Can you work these out from the model? Positions are in its coordinate system, mm. A direction names the side the tool comes from. Give positions to 0.01 mm unless a question says otherwise; leave off trailing zeros. Write each loop counter-clockwise with the first axis right and the second up, starting at its lowest first coordinate (ties: lowest second). Pieces come first, ordered by that corner, then holes.
from build123d import *

# Parameters (mm, degrees)
F0_R     = 45.212
F0_R_2   = 2.032
F1_DEPTH = 6.35
F2_DEPTH = 10.16


with BuildPart() as f1:
    # F0 (on Front) → F1 (new body)
    with BuildSketch(Plane.XZ):
        Circle(F0_R)
        with BuildLine():
            ThreePointArc((37.1053751064, 15.2894918888), (39.3680729638, 7.7930902161), (40.132, 0))
            ThreePointArc((40.132, 0), (39.3680729638, -7.7930902161), (37.1053751064, -15.2894918888))
            ThreePointArc((37.1053751064, -15.2894918888), (34.7553315047, -20.066), (31.7937759398, -24.4894515147))
            ThreePointArc((31.7937759398, -24.4894515147), (20.066, -34.7553315047), (5.3115991666, -39.7789434034))
            ThreePointArc((5.3115991666, -39.7789434034), (0, -40.132), (-5.3115991666, -39.7789434034))
            ThreePointArc((-5.3115991666, -39.7789434034), (-20.066, -34.7553315047), (-31.7937759398, -24.4894515147))
            ThreePointArc((-31.7937759398, -24.4894515147), (-34.7553315047, -20.066), (-37.1053751064, -15.2894918888))
            ThreePointArc((-37.1053751064, -15.2894918888), (-40.132, 0), (-37.1053751064, 15.2894918888))
            ThreePointArc((-37.1053751064, 15.2894918888), (-34.7553315047, 20.066), (-31.7937759398, 24.4894515147))
            ThreePointArc((-31.7937759398, 24.4894515147), (-20.066, 34.7553315047), (-5.3115991666, 39.7789434034))
            ThreePointArc((-5.3115991666, 39.7789434034), (0, 40.132), (5.3115991666, 39.7789434034))
            ThreePointArc((5.3115991666, 39.7789434034), (20.066, 34.7553315047), (31.7937759398, 24.4894515147))
            ThreePointArc((31.7937759398, 24.4894515147), (34.7553315047, 20.066), (37.1053751064, 15.2894918888))
        make_face(mode=Mode.SUBTRACT)
        Polygon((4.2527620829, -7.366), (8.5055241657, 0), (4.2527620829, 7.366), (-4.2527620829, 7.366), (-8.5055241657, 0), (-4.2527620829, -7.366), align=None)
        Circle(F0_R_2, mode=Mode.SUBTRACT)
        with BuildLine():
            Line((1.5875, 35.4173183441), (5.3115991666, 39.7789434034))
            ThreePointArc((5.3115991666, 39.7789434034), (0, 40.132), (-5.3115991666, 39.7789434034))
            Line((-5.3115991666, 39.7789434034), (-1.5875, 35.4173183441))
            Line((-1.5875, 35.4173183441), (-1.5875, 12.7893453464))
            Line((-1.5875, 12.7893453464), (-5.4585231293, 9.4544393942))
            Line((-5.4585231293, 9.4544393942), (5.4585231293, 9.4544393942))
            Line((5.4585231293, 9.4544393942), (1.5875, 12.7893453464))
            Line((1.5875, 12.7893453464), (1.5875, 35.4173183441))
        make_face()
        with BuildLine():
            Line((-29.8785474199, 19.0834745006), (-31.7937759398, 24.4894515147))
            ThreePointArc((-31.7937759398, 24.4894515147), (-34.7553315047, 20.066), (-37.1053751064, 15.2894918888))
            Line((-37.1053751064, 15.2894918888), (-31.4660474199, 16.3338438436))
            Line((-31.4660474199, 16.3338438436), (-11.8696479677, 5.0198573447))
            Line((-11.8696479677, 5.0198573447), (-10.9170462585, 0))
            Line((-10.9170462585, 0), (-5.4585231293, 9.4544393942))
            Line((-5.4585231293, 9.4544393942), (-10.2821479677, 7.7694880017))
            Line((-10.2821479677, 7.7694880017), (-29.8785474199, 19.0834745006))
        make_face()
        with BuildLine():
            ThreePointArc((-37.1053751064, -15.2894918888), (-34.7553315047, -20.066), (-31.7937759398, -24.4894515147))
            Line((-31.7937759398, -24.4894515147), (-29.8785474199, -19.0834745006))
            Line((-29.8785474199, -19.0834745006), (-10.2821479677, -7.7694880017))
            Line((-10.2821479677, -7.7694880017), (-5.4585231293, -9.4544393942))
            Line((-5.4585231293, -9.4544393942), (-10.9170462585, 0))
            Line((-10.9170462585, 0), (-11.8696479677, -5.0198573447))
            Line((-11.8696479677, -5.0198573447), (-31.4660474199, -16.3338438436))
            Line((-31.4660474199, -16.3338438436), (-37.1053751064, -15.2894918888))
        make_face()
        with BuildLine():
            ThreePointArc((-5.3115991666, -39.7789434034), (0, -40.132), (5.3115991666, -39.7789434034))
            Line((5.3115991666, -39.7789434034), (1.5875, -35.4173183441))
            Line((1.5875, -35.4173183441), (1.5875, -12.7893453464))
            Line((1.5875, -12.7893453464), (5.4585231293, -9.4544393942))
            Line((5.4585231293, -9.4544393942), (-5.4585231293, -9.4544393942))
            Line((-5.4585231293, -9.4544393942), (-1.5875, -12.7893453464))
            Line((-1.5875, -12.7893453464), (-1.5875, -35.4173183441))
            Line((-1.5875, -35.4173183441), (-5.3115991666, -39.7789434034))
        make_face()
        with BuildLine():
            ThreePointArc((31.7937759398, -24.4894515147), (34.7553315047, -20.066), (37.1053751064, -15.2894918888))
            Line((37.1053751064, -15.2894918888), (31.4660474199, -16.3338438436))
            Line((31.4660474199, -16.3338438436), (11.8696479677, -5.0198573447))
            Line((11.8696479677, -5.0198573447), (10.9170462585, 0))
            Line((10.9170462585, 0), (5.4585231293, -9.4544393942))
            Line((5.4585231293, -9.4544393942), (10.2821479677, -7.7694880017))
            Line((10.2821479677, -7.7694880017), (29.8785474199, -19.0834745006))
            Line((29.8785474199, -19.0834745006), (31.7937759398, -24.4894515147))
        make_face()
        with BuildLine():
            Line((31.4660474199, 16.3338438436), (37.1053751064, 15.2894918888))
            ThreePointArc((37.1053751064, 15.2894918888), (34.7553315047, 20.066), (31.7937759398, 24.4894515147))
            Line((31.7937759398, 24.4894515147), (29.8785474199, 19.0834745006))
            Line((29.8785474199, 19.0834745006), (10.2821479677, 7.7694880017))
            Line((10.2821479677, 7.7694880017), (5.4585231293, 9.4544393942))
            Line((5.4585231293, 9.4544393942), (10.9170462585, 0))
            Line((10.9170462585, 0), (11.8696479677, 5.0198573447))
            Line((11.8696479677, 5.0198573447), (31.4660474199, 16.3338438436))
        make_face()
        Polygon((-4.2527620829, 7.366), (-5.4585231293, 9.4544393942), (-10.9170462585, 0), (-8.5055241657, 0), align=None)
        Polygon((-10.9170462585, 0), (-5.4585231293, -9.4544393942), (-4.2527620829, -7.366), (-8.5055241657, 0), align=None)
        Polygon((-5.4585231293, -9.4544393942), (5.4585231293, -9.4544393942), (4.2527620829, -7.366), (-4.2527620829, -7.366), align=None)
        Polygon((5.4585231293, -9.4544393942), (10.9170462585, 0), (8.5055241657, 0), (4.2527620829, -7.366), align=None)
        Polygon((8.5055241657, 0), (10.9170462585, 0), (5.4585231293, 9.4544393942), (4.2527620829, 7.366), align=None)
        Polygon((4.2527620829, 7.366), (5.4585231293, 9.4544393942), (-5.4585231293, 9.4544393942), (-4.2527620829, 7.366), align=None)
    extrude(amount=F1_DEPTH)

    # F0 (on Front) → F2 (join)
    with BuildSketch(Plane.XZ):
        Polygon((-10.9170462585, 0), (-5.4585231293, -9.4544393942), (-4.2527620829, -7.366), (-8.5055241657, 0), align=None)
        Polygon((-5.4585231293, -9.4544393942), (5.4585231293, -9.4544393942), (4.2527620829, -7.366), (-4.2527620829, -7.366), align=None)
        Polygon((5.4585231293, -9.4544393942), (10.9170462585, 0), (8.5055241657, 0), (4.2527620829, -7.366), align=None)
        Polygon((8.5055241657, 0), (10.9170462585, 0), (5.4585231293, 9.4544393942), (4.2527620829, 7.366), align=None)
        Polygon((4.2527620829, 7.366), (5.4585231293, 9.4544393942), (-5.4585231293, 9.4544393942), (-4.2527620829, 7.366), align=None)
        Polygon((-4.2527620829, 7.366), (-5.4585231293, 9.4544393942), (-10.9170462585, 0), (-8.5055241657, 0), align=None)
    extrude(amount=F2_DEPTH)


solid = f1.part
(1) Imagine slicing it at B-B, the plane x = 22. Write out the boundary of the cut face in (y, z), plus the area to 3 significant figures.
Returned:
outline: (-6.35, -39.5) - (0, -39.5) - (0, -33.56) - (-6.35, -33.56) - close; (-6.35, -14.53) - (0, -14.53) - (0, -10.87) - (-6.35, -10.87) - close; (-6.35, 10.87) - (0, 10.87) - (0, 14.53) - (-6.35, 14.53) - close; (-6.35, 33.56) - (0, 33.56) - (0, 39.5) - (-6.35, 39.5) - close
area: 122 mm2
(2) If I drill on L1, parallel to Z at x = 0, y = -3; L2, parallel to Z at x = 3, y = -0.25; L3, parallel to Z at x = 23, y = -6.25, over which ranges is the centre line in solid material (lowest first)?
Returned:
L1: z = -45.21 to -2.03, 2.03 to 45.21
L2: z = -45.11 to -37.07, -11.57 to 11.57, 37.07 to 45.11
L3: z = -38.92 to -32.89, -15.11 to -11.45, 11.45 to 15.11, 32.89 to 38.92
(3) Imagine slicing it at A-A, the plane x = 0. Write out the boundary of the cut face in (y, z).
Returned:
outline: (-10.16, -9.45) - (-6.35, -9.45) - (-6.35, -45.21) - (0, -45.21) - (0, -2.03) - (-6.35, -2.03) - (-6.35, -7.37) - (-10.16, -7.37) - close; (-10.16, 7.37) - (-6.35, 7.37) - (-6.35, 2.03) - (0, 2.03) - (0, 45.21) - (-6.35, 45.21) - (-6.35, 9.45) - (-10.16, 9.45) - close
(4) Will these pins go through, and if not, where does the flat tip stop? P1, Ø2, axis at x = 20.5, y = -6.5, coming from the -Z side; P2, Ø3, axis at y = -4, z = -29, coming from the -X side; P3, Ø1.9, axis at y = -4, z = 20.5, coming from the -X side.
Returned:
P1: stops at z = -40.79
P2: stops at x = -35.89
P3: stops at x = -40.77
(5) Imagine slicing it at C-C, the plane z = -38. Write out the boundary of the cut face in (x, y), plus the area to 3 significant figures.
Returned:
outline: (-24.5, -6.35) - (-12.91, -6.35) - (-12.91, 0) - (-24.5, 0) - close; (-3.79, -6.35) - (3.79, -6.35) - (3.79, 0) - (-3.79, 0) - close; (12.91, -6.35) - (24.5, -6.35) - (24.5, 0) - (12.91, 0) - close
area: 195 mm2
(6) Imagine slicing it at D-D, the plane x = -27. Write out the boundary of the cut face in (y, z).
Returned:
outline: (-6.35, -36.26) - (0, -36.26) - (0, -29.69) - (-6.35, -29.69) - close; (-6.35, -17.42) - (0, -17.42) - (0, -13.76) - (-6.35, -13.76) - close; (-6.35, 13.76) - (0, 13.76) - (0, 17.42) - (-6.35, 17.42) - close; (-6.35, 29.69) - (0, 29.69) - (0, 36.26) - (-6.35, 36.26) - close
(7) For faces 1 (the face through (-30.85, -3.13, -21.82)), 2 (the face through (8.15, -8.23, -4.79)), 3 (the face through (-8.226, -8.228, -4.661)), which set-ups out of +Z, -Z, +X, -X, +Y, -Y let a thin tool reach every point of the face, with its end or its side?
Returned:
face 1: +Y, -Y
face 2: -Z, +X, -Y
face 3: -Z, -X, -Y
